from build123d import *

# Parameters (mm, degrees)
F1_DEPTH      = 44.45
F4_ANGLE_BACK = 90
F4_ANGLE      = 180
F10_D         = 9.525


# Not quite as in the source:
# - a pattern or mirror of a feature is missing from the dataset's text; its kind, count and spacing are read off the source's solid


with BuildPart() as f1:
    # F0 (on Top) → F1 (new body)
    with BuildSketch(Plane.XY):
        with BuildLine():
            Line((-31.75, 63.5), (-31.75, 0))
            ThreePointArc((-31.75, 0), (0, -31.75), (31.75, 0))
            Line((31.75, 0), (31.75, 63.5))
            ThreePointArc((31.75, 63.5), (0, 95.25), (-31.75, 63.5))
        make_face()
    extrude(amount=F1_DEPTH)

    # F3 (on Right) → F4 (revolve, cut)
    with BuildSketch(Plane.YZ, mode=Mode.PRIVATE) as f4_sk:
        Polygon((-31.75, 0), (-12.7, 44.45), (-31.75, 44.45), align=None)
    f4 = revolve(f4_sk.sketch.rotate(Axis((0, 19.05, 31.5998233855), (0, 0, 1)), -F4_ANGLE_BACK), axis=Axis((0, 19.05, 31.5998233855), (0, 0, 1)), revolution_arc=F4_ANGLE, mode=Mode.SUBTRACT)

    # F4_copies: F4 across plane
    add(f4.mirror(Plane(origin=(4e-05, 31.750043, -6e-06), x_dir=(1, -1e-06, 0), z_dir=(1e-06, 1, 0))), mode=Mode.SUBTRACT)

    # F5 (on Right) → F6 (revolve)
    with BuildSketch(Plane.YZ):
        Polygon((-9.525, 57.15), (-12.7, 44.45), (0, 44.45), (0, 57.15), align=None)
    f6 = revolve(axis=Axis((0, 0, 50.8), (0, 0, -1)))

    # F6_copies: F6 across plane
    add(f6.mirror(Plane.ZX.offset(31.75)))

    # F7 (on Right) → F8 (revolve, cut)
    with BuildSketch(Plane.YZ):
        Polygon((20.6375, 0), (31.75, 0), (31.75, 44.45), (15.875, 44.45), align=None)
    revolve(axis=Axis((0, 31.75, 22.225), (0, 0, 1)), mode=Mode.SUBTRACT)

    # F10 (through all)
    with Locations(Plane.XY.offset(57.15)):
        with Locations((0, 0), (0, 63.5)):
            Hole(F10_D / 2)


solid = f1.part
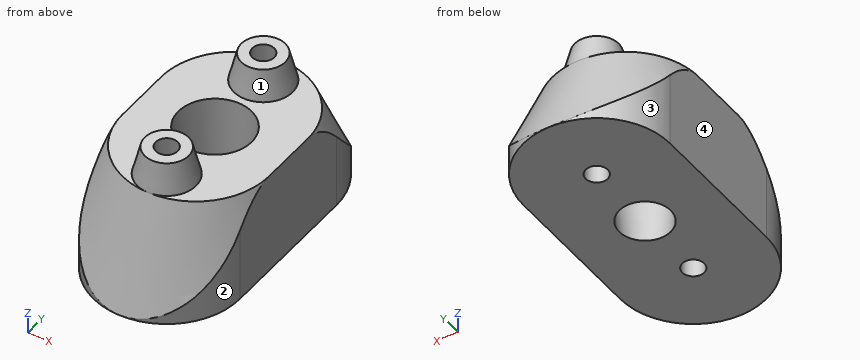
Read the model definition and answer for the solid it produces. Units are mm, in the model's axes. Face numbers are marked on the shaded views. Round coordinates to 2 decimals unless told otherwise and drop trailing zeros. Loops run counter-clockwise (first coordinate to the right, second up) from the corner with the lowest first, then second, coordinate; pieces in that order, holes last. Notation, with made-up numbers: (-33.5, 32.5) - (-13.5, 32.5) arc R34 cw to (-13.5, 65.5) - close; hole circle Ø11 at (24, -7). An arc over 180 degrees is marked (long way). One line per question, with ' | ' between items. Start each with the question number.
Q1. Find the intervals of material crossed by L1, parallel to X at y = 63, z = 19; L2, parallel to Y at x = 0, z = 42; L3, parallel to Y at x = 0, z = 25, in increasing order.
Q2. Section A-A on z = 16 is taken. Count the separate pieces of the cut face and the enclosed holes in it, plus the area to 3 significant figures.
Q3. For a pull along Y with two mould halves and no side action, classify the marked faces 1, 2, 3 and 4 as +Y half, -Y half, draft (parallel to the pull), parting line (faces both ways), or undercut.
Q4. Flat-ended cylindrical pins translate along their axes: pin 1 (12.5 mm diameter, centred on x = 0, y = 63.5, fed in from -Z); pin 2 (5 mm diameter, centred on x = 18.5, y = 65, fed in from +Z); pin 3 (1.5 mm diameter, centred on x = 11.5, y = 81, fed in from +Z). Find the tip coordinate at first contact, or state that the pin passes through.
Q5. Section D-D on z = 49.5 is taken. Give the vertices of the cut face in (x, y) (1 decimal), plus the area to 3 significant figures.
Established:
1) L1: -31.75 to -4.74, 4.74 to 31.75 | L2: -13.75 to -4.76, 4.76 to 16.14, 47.36 to 58.74, 68.26 to 77.25 | L3: -21.04 to -4.76, 4.76 to 17.96, 45.54 to 58.74, 68.26 to 84.54
2) separate pieces: 1 | enclosed holes: 3 | area: 5,960 mm²
3) face 1: undercut | face 2: -Y half | face 3: +Y half | face 4: draft
4) pin 1: z = 0 | pin 2: z = 44.45 | pin 3: z = 30.88
5) outline: circle Ø22.9 at (0, 0); circle Ø22.9 at (0, 63.5); hole circle Ø9.5 at (0, 0); hole circle Ø9.5 at (0, 63.5) | area: 679 mm²
